Drawing for the job (mm, zero at the part's lowest x, y, z). Give positions to 0.01 mm unless a question says otherwise; leave off trailing zeros. Order: outer loops, then holes, each group sorted by start corner. A loop starts at its lowest first (then second) coordinate and runs counter-clockwise, first axis right, second up. Notation, with made-up numbers: (-27.5, 81.5) - (-11.5, 81.5) arc R27 cw to (-11.5, 112.5) - close; hole circle Ø1 at (62, 32.25). An arc over 180 degrees is marked (long way). Use a Markdown table: item, result.
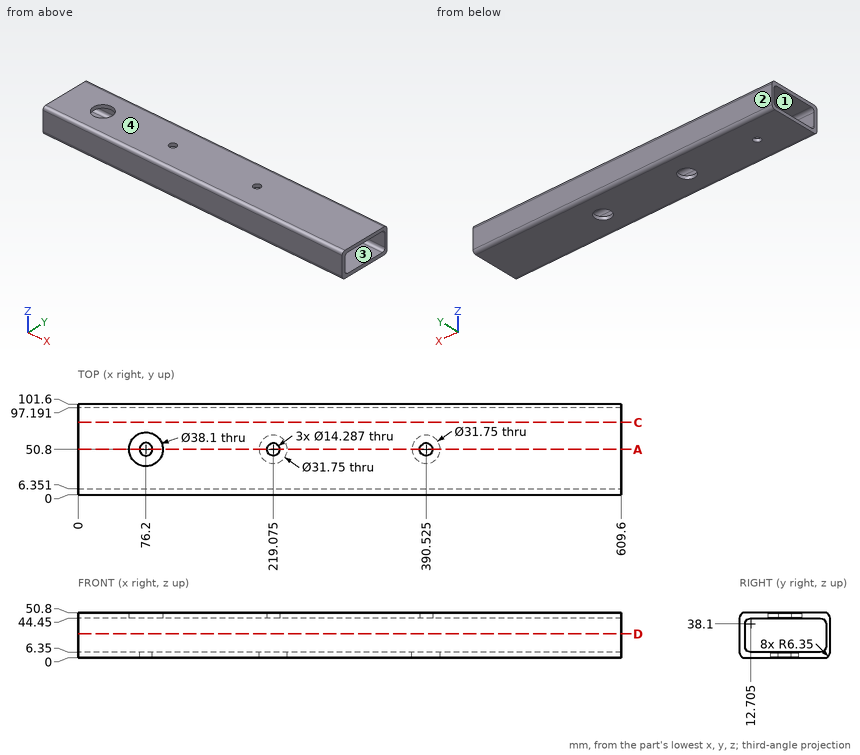
1) Slice it at C-C (y = 81). Write the cut outline in (x, z).
Computed:
| item | result |
|---|---|
| outline | (0, 0) - (609.6, 0) - (609.6, 6.35) - (0, 6.35) - close; (0, 44.45) - (609.6, 44.45) - (609.6, 50.8) - (0, 50.8) - close |
2) Two-plate mould, pull along Z, no slides. Class the marked faces 1, 2, 3 and 4: +Z half, -Z half, draft (parallel to the pull), parting line (faces both ways), or undercut.
Computed:
| item | result |
|---|---|
| face 1 | undercut |
| face 2 | draft |
| face 3 | undercut |
| face 4 | +Z half |
3) Wall check: line 1 (X direction, y = 51.5, z = 48) (1 decimal); line 2 (X direction, y = 50, z = 4); line 3 (Z direction, x = 128, y = 71). Give the ranges that are in metal, low to high. Write a range as from..to.
Computed:
| item | result |
|---|---|
| line 1 | x = 0..57.2, 95.2..212, 226.2..383.4, 397.6..609.6 |
| line 2 | x = 0..69.1, 83.3..203.22, 234.93..374.67, 406.38..609.6 |
| line 3 | z = 0..6.35, 44.45..50.8 |
4) Slice it at A-A (y = 50.8). State how many separate pieces and enclosed holes the cut face has.
Computed:
| item | result |
|---|---|
| separate pieces | 8 |
| enclosed holes | 0 |
5) Slice it at D-D (z = 27). Write the cut outline in (x, y).
Computed:
| item | result |
|---|---|
| outline | (0, 0) - (609.6, 0) - (609.6, 6.35) - (0, 6.35) - close; (0, 97.19) - (609.6, 97.19) - (609.6, 101.6) - (0, 101.6) - close |
6) Pin check, flat tips, straight feed: P1, Ø23, axis at x = 390.525, y = 50.8, coming from the +Z side; P2, Ø18.5, axis at x = 219.075, y = 50.8, coming from the -Z side. Stop position of each tip, or through.
Computed:
| item | result |
|---|---|
| P1 | stops at z = 50.8 |
| P2 | stops at z = 44.45 |
